from build123d import *

# Parameters (mm, degrees)
F7_DEPTH       = 101.6
F2_DEPTH       = 25.4
F2_DEPTH_BACK  = 25.4
F4_D           = 12.7
F4_ON_F1_D     = 12.7
F4_ON_F1_DEPTH = 25.401
F5_D           = 12.7
F6_R           = 1.27


with BuildPart() as f7:
    # F0 (on Front) → F7 (new body)
    with BuildSketch(Plane.XZ):
        with BuildLine():
            Line((-22.225, -25.4), (22.225, -25.4))
            ThreePointArc((22.225, -25.4), (24.4700640303, -24.4700640303), (25.4, -22.225))
            Line((25.4, -22.225), (25.4, 22.225))
            ThreePointArc((25.4, 22.225), (24.4700640303, 24.4700640303), (22.225, 25.4))
            Line((22.225, 25.4), (-22.225, 25.4))
            ThreePointArc((-22.225, 25.4), (-24.4700640303, 24.4700640303), (-25.4, 22.225))
            Line((-25.4, 22.225), (-25.4, -22.225))
            ThreePointArc((-25.4, -22.225), (-24.4700640303, -24.4700640303), (-22.225, -25.4))
        make_face()
        with BuildLine():
            ThreePointArc((20.6375, -17.4625), (19.7075640303, -19.7075640303), (17.4625, -20.6375))
            Line((17.4625, -20.6375), (-17.4625, -20.6375))
            ThreePointArc((-17.4625, -20.6375), (-19.7075640303, -19.7075640303), (-20.6375, -17.4625))
            Line((-20.6375, -17.4625), (-20.6375, 17.4625))
            ThreePointArc((-20.6375, 17.4625), (-19.7075640303, 19.7075640303), (-17.4625, 20.6375))
            Line((-17.4625, 20.6375), (17.4625, 20.6375))
            ThreePointArc((17.4625, 20.6375), (19.7075640303, 19.7075640303), (20.6375, 17.4625))
            Line((20.6375, 17.4625), (20.6375, -17.4625))
        make_face(mode=Mode.SUBTRACT)
    extrude(amount=F7_DEPTH)

    # F1 (on Top) → F2 (cut, two sides)
    with BuildSketch(Plane.XY) as f2_sk:
        Polygon((-15.875, -63.5), (-15.875, 0), (-37.8918275237, 0), (-37.8918275237, -101.6), (-20.6375, -101.6), (-15.875, -101.6), align=None)
    extrude(amount=-F2_DEPTH, mode=Mode.SUBTRACT)
    extrude(f2_sk.sketch, amount=F2_DEPTH_BACK, mode=Mode.SUBTRACT)

    # F4 (through all)
    with Locations(Plane(origin=(0, 0, 0), x_dir=(0, 1, 0), z_dir=(-1, 0, 0))):
        with Locations((-82.55, 0)):
            Hole(F4_D / 2)

    # F4 on F1 (through all, one way)
    with BuildSketch(Plane(origin=(0, 0, 0), x_dir=(1, 0, 0), z_dir=(0, 0, -1))):
        with Locations((0, 19.05)):
            Circle(F4_ON_F1_D / 2)
    extrude(amount=-F4_ON_F1_DEPTH, mode=Mode.SUBTRACT)

    # F5 (through all)
    with Locations(Plane.XY):
        with Locations((0, -19.05)):
            Hole(F5_D / 2)

    # F6
    f6_edges = [f7.edges().sort_by_distance(p)[0] for p in [
        (25.4, -101.6, 0),
    ]]
    fillet(f6_edges, radius=F6_R)


solid = f7.part
Check sheet for the modelled part. Datum: model origin and axes. Units: mm. A direction names the side the tool comes from. Give positions to 0.01 mm unless a question says otherwise; leave off trailing zeros. Write each loop counter-clockwise with the first axis right and the second up, starting at its lowest first coordinate (ties: lowest second). Pieces come first, ordered by that corner, then holes. Notation, with made-up numbers: (88.25, 53) -> (108.25, 53) arc R30 cw to (108.25, 82) -> close; hole circle Ø2 at (-1, 72). An arc over 180 degrees is marked (long way). One line per item, written item: value. Start each with the question number.
Item 1: Gauge pin test, flat ends, axial feed: pin 1 (17.5 mm diameter, centred on y = -45.5, z = 3.5, fed in from -X); pin 2 (11.5 mm diameter, centred on x = 0, y = -19.05, fed in from -Z); pin 3 (1.5 mm diameter, centred on y = -44.5, z = 18, fed in from -X). Record the tip position at first contact, or that the pin passes through.
Item 2: Material ranges on probe 1 along Z at (x, y) = (-3.5, -10); probe 2 along X at (y, z) = (-19, -21) (3 decimals); probe 3 along Y at (x, z) = (0, 23.65), recorded low to high. Write a range as from..to.
Item 3: Section check A-A on y = -19.05. State how many separate pieces and enclosed holes the cut face has, then the cut area to 3 significant figures.
Item 4: Tool access check on faces 1 (the flat face through (1, -50, -20.638)), 2 (the cylindrical face through (24.45, -49.46, -24.49)). Record the directions out of +Z, -Z, +X, -X, +Y, -Y that give a thin tool (end or side, any length) a straight path to the whole face; none if there is none.
Item 5: Section check C-C on z = 0. Record the cut outline in (x, y), then the cut area to 3 significant figures.
Item 6: Section check B-B on x = -9.5. Record the cut outline in (y, z), then the cut area to 3 significant figures.
Item 7: Draft check along X on faces 3 (the cylindrical face through (1.38, -25.25, -23.05)), 4 (the flat face through (3, -49, -25.4)), 5 (the flat face through (-15.875, -52, -23)). Enter one of: +X half, -X half, draft (parallel to the pull), parting line (faces both ways), or undercut.
Results list:
1. pin 1: x = 20.64
1. pin 2: through
1. pin 3: x = 20.36
2. probe 1: -25.4..-20.64, 20.64..25.4
2. probe 2: -15.875..-6.35, 6.35..25.4
2. probe 3: -101.6..-25.4, -12.7..0
3. separate pieces: 3
3. enclosed holes: 0
3. area: 469 mm²
4. face 1: -X, +Y, -Y
4. face 2: -Z, +X, +Y, -Y
5. outline: (20.64, -101.6) -> (24.13, -101.6) arc R1.27 ccw to (25.4, -100.33) -> (25.4, -88.9) -> (20.64, -88.9) -> close; (20.64, -76.2) -> (25.4, -76.2) -> (25.4, 0) -> (20.64, 0) -> close
5. area: 423 mm²
6. outline: (-101.6, -24.13) arc R1.27 ccw to (-100.33, -25.4) -> (0, -25.4) -> (0, -20.64) -> (-101.6, -20.64) -> close; (-101.6, 20.64) -> (0, 20.64) -> (0, 25.4) -> (-100.33, 25.4) arc R1.27 ccw to (-101.6, 24.13) -> close
6. area: 967 mm²
7. face 3: undercut
7. face 4: draft
7. face 5: -X half
